from build123d import *

# Parameters (mm, degrees)
SKETCH_1_R      = 7.5
SKETCH_1_R_2    = 1.6
SKETCH_1_W      = 15
SKETCH_1_H      = 40
EXTRUDE_1_DEPTH = 3
FILLET_1_R      = 3


with BuildPart() as part:
    # 草图1 → 凸台-拉伸1 (new body)
    with BuildSketch(Plane(origin=(0, 0, 0), x_dir=(1, 0, 0), z_dir=(0, 1, 0))):
        with BuildLine():
            Line((-12.4, 320), (-12.4, 0))
            Line((-12.4, 0), (12.4, 0))
            Line((12.4, 0), (12.4, 320))
            ThreePointArc((12.4, 320), (0, 332.4), (-12.4, 320))
        make_face()
        with Locations(Location((0, 320, 0), (0, 0, 270))):
            Circle(SKETCH_1_R, mode=Mode.SUBTRACT)
        with Locations(Location((10, 3, 0), (0, 0, 270))):
            Circle(SKETCH_1_R_2, mode=Mode.SUBTRACT)
        with Locations(Location((-10, 3, 0), (0, 0, 90))):
            Circle(SKETCH_1_R_2, mode=Mode.SUBTRACT)
        with Locations((0, 235)):
            Rectangle(SKETCH_1_W, SKETCH_1_H, mode=Mode.SUBTRACT)
        with Locations((0, 285)):
            Rectangle(SKETCH_1_W, SKETCH_1_H, mode=Mode.SUBTRACT)
        with Locations((0, 185)):
            Rectangle(SKETCH_1_W, SKETCH_1_H, mode=Mode.SUBTRACT)
        with Locations((0, 135)):
            Rectangle(SKETCH_1_W, SKETCH_1_H, mode=Mode.SUBTRACT)
        with Locations((0, 85)):
            Rectangle(SKETCH_1_W, SKETCH_1_H, mode=Mode.SUBTRACT)
        with Locations((0, 35)):
            Rectangle(SKETCH_1_W, SKETCH_1_H, mode=Mode.SUBTRACT)
    extrude(amount=EXTRUDE_1_DEPTH)

    # 圆角1
    fillet_1_edges = [part.edges().sort_by_distance(p)[0] for p in [
        (7.5, 1.5, -265),
        (7.5, 1.5, -305),
        (-7.5, 1.5, -305),
        (-7.5, 1.5, -265),
        (-7.5, 1.5, -215),
        (7.5, 1.5, -215),
        (7.5, 1.5, -255),
        (-7.5, 1.5, -255),
        (-7.5, 1.5, -165),
        (7.5, 1.5, -165),
        (7.5, 1.5, -205),
        (-7.5, 1.5, -205),
        (-7.5, 1.5, -115),
        (7.5, 1.5, -115),
        (7.5, 1.5, -155),
        (-7.5, 1.5, -155),
        (-7.5, 1.5, -65),
        (7.5, 1.5, -65),
        (7.5, 1.5, -105),
        (-7.5, 1.5, -105),
        (-7.5, 1.5, -15),
        (7.5, 1.5, -15),
        (7.5, 1.5, -55),
        (-7.5, 1.5, -55),
    ]]
    fillet(fillet_1_edges, radius=FILLET_1_R)


solid = part.part
The listing builds one solid part. Answer for the finished solid, in the listing's coordinates (mm). Coordinates: 2 decimals unless noted, no trailing zeros. Answer in a Markdown table with one row per item. Add a question column.
Item 1: Find the intervals of material crossed by L1, parallel to X at y = 2.35, z = -3; L2, parallel to X at y = 2.3, z = -320; L3, parallel to X at y = 2.3, z = -266, in increasing order. Write a range as from..to.
Item 2: Determine the mould class of faces 1 (the face through (-8, 0, -169)), 2 (the face through (0.273, 1.479, -332.397)), 3 (the face through (5.1, 1.5, -325.5)) for opening direction Z: +Z half, -Z half, draft (parallel to the pull), parting line (faces both ways), or undercut.
Item 3: Each of these flat-tipped pins is pushed along its axis until it touches: P1, Ø0.9, axis at x = -0.5, y = 1.5, coming from the +Z side; P2, Ø1.9, axis at x = -10, z = -3, coming from the -Y side; P3, Ø0.9, axis at x = 1.5, y = 1, coming from the -Z side. Where does it stop, or does it pass through?
Item 4: Find section A-A (x = 0). State how many separate pieces and enclosed holes the cut face has, then the cut area to 3 significant figures.
Result set:
| question | item | result |
|---|---|---|
| 1 | L1 | x = -12.4..-11.6, -8.4..8.4, 11.6..12.4 |
| 1 | L2 | x = -12.4..-7.5, 7.5..12.4 |
| 1 | L3 | x = -12.4..-6.74, 6.74..12.4 |
| 2 | face 1 | draft |
| 2 | face 2 | -Z half |
| 2 | face 3 | undercut |
| 3 | P1 | stops at z = 0 |
| 3 | P2 | passes through |
| 3 | P3 | stops at z = -332.36 |
| 4 | separate pieces | 8 |
| 4 | enclosed holes | 0 |
| 4 | area | 232 mm² |
